The model under review builds one solid part; all positions refer to its coordinate system, in mm. Face numbers are marked on the shaded views. A direction names the side the tool comes from. Give positions to 0.01 mm unless a question says otherwise; leave off trailing zeros. Write each loop counter-clockwise with the first axis right and the second up, starting at its lowest first coordinate (ties: lowest second). Pieces come first, ordered by that corner, then holes. Notation, with made-up numbers: M 52.25,44.25 L 90.25,44.25 A15 cw 90.25,60.25 Z; hole C 49,55.25 d3. An arc over 180 degrees is marked long. Write each question's results on one line, items separated by ' | '. Start each with the question number.
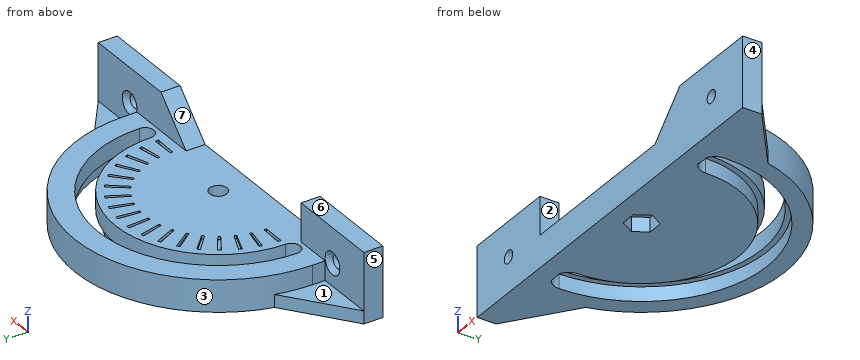
from build123d import *

# Parameters (mm, degrees)
SKETCH1_R                = 2.75
BOSS_EXTRUDE1_DEPTH      = 10
CUT_EXTRUDE1_DEPTH       = 4.5
CUT_EXTRUDE2_DEPTH       = 1
CIRPATTERN1_COUNT        = 18
CIRPATTERN1_ANGLE        = 180
SKETCH4_W                = 30
SKETCH4_H                = 22
SKETCH4_R                = 2
BOSS_EXTRUDE2_DEPTH      = 6
CHAMFER3_SIZE            = 12
BOSS_EXTRUDE3_DEPTH      = 4
CHAMFER4_SIZE            = 1.5
CHAMFER4_OF_MIRROR1_SIZE = 1.5


with BuildPart() as part:
    # Sketch1 → Boss-Extrude1 (new body)
    with BuildSketch(Plane.XY):
        with BuildLine():
            Line((-45, 0), (-45, -10))
            Line((-45, -10), (45, -10))
            Line((45, -10), (45, 0))
            ThreePointArc((45, 0), (0, 45), (-45, 0))
        make_face()
        Circle(SKETCH1_R, mode=Mode.SUBTRACT)
        with BuildLine():
            ThreePointArc((-32.25, 0), (0, 32.25), (32.25, 0))
            ThreePointArc((32.25, 0), (35, -2.75), (37.75, 0))
            ThreePointArc((37.75, 0), (0, 37.75), (-37.75, 0))
            ThreePointArc((-37.75, 0), (-35, -2.75), (-32.25, 0))
        make_face(mode=Mode.SUBTRACT)
    extrude(amount=BOSS_EXTRUDE1_DEPTH)

    # Sketch2 → Cut-Extrude1 (cut)
    with BuildSketch(Plane(origin=(0, 0, 0), x_dir=(-1, 0, 0), z_dir=(0, 0, -1))):
        Polygon((4.907477288, 0), (2.453738644, -4.25), (-2.453738644, -4.25), (-4.907477288, 0), (-2.453738644, 4.25), (2.453738644, 4.25), align=None)
        with BuildLine():
            ThreePointArc((-30.5, 0), (0, 30.5), (30.5, 0))
            ThreePointArc((30.5, 0), (35, -4.5), (39.5, 0))
            ThreePointArc((39.5, 0), (0, 39.5), (-39.5, 0))
            ThreePointArc((-39.5, 0), (-35, -4.5), (-30.5, 0))
        make_face()
    extrude(amount=-CUT_EXTRUDE1_DEPTH, mode=Mode.SUBTRACT)

    # Sketch3 → Cut-Extrude2 (cut)
    with BuildSketch(Plane.XY.offset(10)):
        with BuildLine():
            Line((-29.983333333, 0.999861101), (-22.987222222, 0.766560178))
            ThreePointArc((-22.987222222, 0.766560178), (-22.996805334, 0.383333333), (-23, 0))
            Line((-23, 0), (-30, 0))
            ThreePointArc((-30, 0), (-29.995833044, 0.5), (-29.983333333, 0.999861101))
        make_face()
    cut_extrude2 = extrude(amount=-CUT_EXTRUDE2_DEPTH, mode=Mode.SUBTRACT)

    # CirPattern1: Cut-Extrude2 ×18 about axis
    cirpattern1_axis = Axis((0, 0, 0), (0, 0, -1))
    for i in range(1, CIRPATTERN1_COUNT):
        add(cut_extrude2.rotate(cirpattern1_axis, i * CIRPATTERN1_ANGLE / (CIRPATTERN1_COUNT - 1)), mode=Mode.SUBTRACT)

    # Sketch4 → Boss-Extrude2 (add)
    with BuildSketch(Plane.XZ.offset(10)):
        with Locations((48.5, 11)):
            Rectangle(SKETCH4_W, SKETCH4_H)
        with Locations(Location((48.5, 11, 0), (0, 0, 270))):
            Circle(SKETCH4_R, mode=Mode.SUBTRACT)
    boss_extrude2 = extrude(amount=-BOSS_EXTRUDE2_DEPTH)

    # Chamfer3
    chamfer3_edges = [part.edges().sort_by_distance(p)[0] for p in [
        (33.5, -7, 10),
    ]]
    chamfer(chamfer3_edges, length=CHAMFER3_SIZE - 0.0001)  # a hair under: the kernel refuses the full size

    # Sketch5 → Boss-Extrude3 (add)
    with BuildSketch(Plane(origin=(0, 0, 0), x_dir=(-1, 0, 0), z_dir=(0, 0, -1))):
        Polygon((-63.5, -4), (-43.634848459, 11), (-43.634848459, -4), align=None)
    boss_extrude3 = extrude(amount=-BOSS_EXTRUDE3_DEPTH)

    # Chamfer4
    chamfer4_edges = [part.edges().sort_by_distance(p)[0] for p in [
        (48.5, -4, 13),
    ]]
    chamfer(chamfer4_edges, length=CHAMFER4_SIZE)

    # Mirror1: Boss-Extrude2, Boss-Extrude3 across plane
    add(boss_extrude2.mirror(Plane(origin=(0, 0, 0), x_dir=(0, 0, 1), z_dir=(1, 0, 0))))
    add(boss_extrude3.mirror(Plane(origin=(0, 0, 0), x_dir=(0, 0, 1), z_dir=(1, 0, 0))))

    # Chamfer4 of Mirror1
    chamfer4_of_mirror1_edges = [part.edges().sort_by_distance(p)[0] for p in [
        (-48.5, -4, 13),
    ]]
    chamfer(chamfer4_of_mirror1_edges, length=CHAMFER4_OF_MIRROR1_SIZE)


solid = part.part
(1) Add section B-B (z = 19.5). State the section outline as (x, y) points.
(2) Add section C-C (x = 35). State the section outline as (y, z) points, then the cut area to 3 significant figures.
(3) Add section A-A (x = 0). State the section outline as (y, z) points, then the cut area to 3 significant figures.
(4) Add section D-D (x = -48.5). State the section outline as (y, z) points, then the cut area to 3 significant figures.
(5) Clearance check with flat-ended pins moving along their axes: P1, Ø1.2, axis at y = -2.5, z = 6.5, coming from the +X side; P2, Ø1.6, axis at x = 27, y = 5, coming from the +Z side; P3, Ø1.8, axis at x = 36, z = 2.5, coming from the +Y side; P4, Ø2.5, axis at x = 48.5, z = 11, coming from the -Y side. State where each tip first meets the part, or that it passes through.
(6) Wall thickness on L1, parallel to X at y = 26, z = 6; L2, parallel to Z at x = -48.5, y = -7.2; L3, parallel to X at y = 2, z = 1.25: over which ranges is each line inside the solid? List them lowest first.
(7) Machinability: for the marked faces 1, 2 and 3, which of the approach directions +Z, -Z, +X, -X, +Y, -Y give a long, thin tool a straight path to every point of the face, cutting with its end or side? Answer none if there is none.
(8) Draft analysis for pull direction X (two halves, no side actions). For the marked faces 4, 5, 6 and 7, state which applies: pulls with the +X half, pulls with the -X half, needs draft (parallel to the pull), parting line crosses it, or undercut.
Calculated:
1) outline: M -63.5,-10 L -33.5,-10 L -33.5,-4 L -63.5,-4 Z; M 31,-10 L 63.5,-10 L 63.5,-4 L 31,-4 Z
2) outline: M -10,0 L -4,0 L -4,4.5 L -2.75,4.5 L -2.75,10 L -4,10 L -4,22 L -10,22 Z; M 14.14,4.5 L 18.31,4.5 L 18.31,0 L 28.28,0 L 28.28,10 L 14.14,10 Z | area: 262 mm²
3) outline: M -10,0 L -4.25,0 L -4.25,4.5 L -2.75,4.5 L -2.75,10 L -10,10 Z; M 2.75,4.5 L 4.25,4.5 L 4.25,0 L 30.5,0 L 30.5,4.5 L 32.25,4.5 L 32.25,10 L 2.75,10 Z; M 37.75,4.5 L 39.5,4.5 L 39.5,0 L 45,0 L 45,10 L 37.75,10 Z | area: 411 mm²
4) outline: M -10,0 L 7.33,0 L 7.33,4 L -4,4 L -4,7.5 L -5.5,9 L -10,9 Z; M -10,13 L -5.5,13 L -4,14.5 L -4,22 L -10,22 Z | area: 151 mm²
5) P1: stops at x = 45 | P2: stops at z = 10 | P3: stops at y = 28.16 | P4: passes through
6) L1: x = -36.73 to -27.37, -19.08 to 19.08, 27.37 to 36.73 | L2: z = 0 to 9, 13 to 22 | L3: x = -55.55 to -39.45, -30.43 to -3.75, 3.75 to 30.43, 39.45 to 55.55
7) face 1: +Z, -X, +Y | face 2: +Z, +Y, -Y | face 3: +Z, +Y
8) face 4: pulls with the +X half | face 5: pulls with the -X half | face 6: needs draft | face 7: undercut
